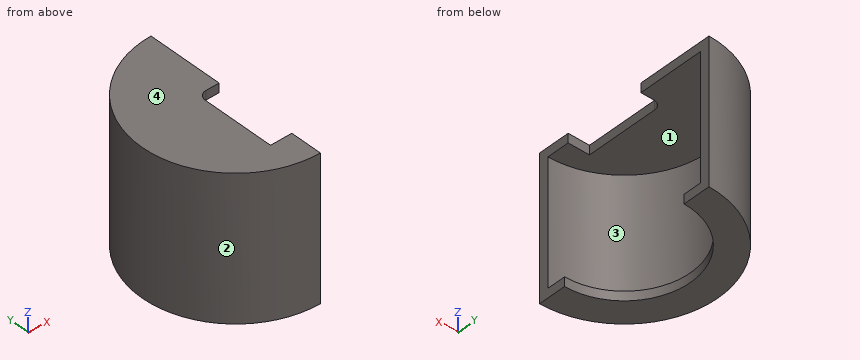
```python
from build123d import *

# Parameters (mm, degrees)
BOSS_EXTRU_1_DEPTH      = 34
BOSS_EXTRU_2_DEPTH      = 5
BOSS_EXTRU_3_DEPTH      = 5
ENL_V_MAT_EXTRU_1_DEPTH = 10


with BuildPart() as part:
    # Esquisse1 → Boss.-Extru.1 (new body, symmetric)
    with BuildSketch(Plane.XY):
        with BuildLine():
            Line((0, 51), (0, 46))
            ThreePointArc((0, 46), (-46, 0), (0, -46))
            Line((0, -46), (0, -51))
            ThreePointArc((0, -51), (-51, 0), (0, 51))
        make_face()
    extrude(amount=BOSS_EXTRU_1_DEPTH, both=True)

    # Esquisse2 → Boss.-Extru.2 (add)
    with BuildSketch(Plane.XY.offset(34)):
        with BuildLine():
            Line((0, 51), (0, -51))
            ThreePointArc((0, -51), (-51, 0), (0, 51))
        make_face()
    extrude(amount=BOSS_EXTRU_2_DEPTH)

    # Esquisse3 → Boss.-Extru.3 (add)
    with BuildSketch(Plane(origin=(0, 0, -34), x_dir=(-1, 0, 0), z_dir=(0, 0, -1))):
        with BuildLine():
            Line((0, 51), (0, 36))
            ThreePointArc((0, 36), (36, 0), (0, -36))
            Line((0, -36), (0, -51))
            ThreePointArc((0, -51), (51, 0), (0, 51))
        make_face()
    extrude(amount=BOSS_EXTRU_3_DEPTH)

    # Esquisse4 → Enlèv. mat.-Extru.1 (cut)
    with BuildSketch(Plane.XY.offset(39)):
        with BuildLine():
            Line((-11.59999996, 5.499999956), (-11.59999996, -2))
            Line((-11.59999996, -2), (-0.788986692, -2))
            ThreePointArc((-0.788986692, -2), (-2.112167134, 0.40155946), (0, 2.15))
            Line((0, 2.15), (0, 10.000000044))
            Line((0, 10.000000044), (-7.099999871, 10.000000044))
            ThreePointArc((-7.099999871, 10.000000044), (-10.281980449, 8.681980534), (-11.59999996, 5.499999956))
        make_face()
        with BuildLine():
            ThreePointArc((0, 2.15), (-2.112167134, 0.40155946), (-0.788986692, -2))
            Line((-0.788986692, -2), (0, -2))
            Line((0, -2), (0, 2.15))
        make_face()
        with BuildLine():
            Line((0, -2), (-0.788986692, -2))
            ThreePointArc((-0.788986692, -2), (-0.40155946, -2.112167134), (0, -2.15))
            Line((0, -2.15), (0, -2))
        make_face()
        with BuildLine():
            Line((0, 2.15), (0, -2))
            Line((0, -2), (0.788986692, -2))
            ThreePointArc((0.788986692, -2), (1.77747312, -1.209582286), (2.15, 0))
            ThreePointArc((2.15, 0), (1.52027958, 1.52027958), (0, 2.15))
        make_face()
        with BuildLine():
            Line((0.788986692, -2), (0, -2))
            Line((0, -2), (0, -2.15))
            ThreePointArc((0, -2.15), (0.40155946, -2.112167134), (0.788986692, -2))
        make_face()
        with BuildLine():
            Line((-0.788986692, -2), (-11.59999996, -2))
            Line((-11.59999996, -2), (-11.59999996, -33.8))
            Line((-11.59999996, -33.8), (0, -33.8))
            Line((0, -33.8), (0, -2.15))
            ThreePointArc((0, -2.15), (-0.40155946, -2.112167134), (-0.788986692, -2))
        make_face()
    extrude(amount=-ENL_V_MAT_EXTRU_1_DEPTH, mode=Mode.SUBTRACT)


solid = part.part
```
Model file for the job. Use its own axes, mm. Face numbers are marked on the shaded views. Give positions to 0.01 mm unless a question says otherwise; leave off trailing zeros. Loops run counter-clockwise (first coordinate to the right, second up) from the corner with the lowest first, then second, coordinate; pieces in that order, holes last. Notation, with made-up numbers: (48, -33) -> (57, -33) arc R10 ccw to (57, -28) -> close; hole circle Ø3 at (-21, 54.5). An arc over 180 degrees is marked (long way). Write each question's results on one line, items separated by ' | '.
(1) Cut at A-A on y = 31. List the corners of the cut face in (x, z), and give its area (3 significant figures).
Geometry results:
outline: (-40.5, -39) -> (-18.3, -39) -> (-18.3, -34) -> (-33.99, -34) -> (-33.99, 34) -> (0, 34) -> (0, 39) -> (-40.5, 39) -> close | area: 756 mm²
(2) Cut at C-C on z = -7. List the corners of the cut face in (x, y).
Geometry results:
outline: (0, -51) -> (0, -46) arc R46 cw to (0, 46) -> (0, 51) arc R51 ccw to start
(3) Probe line 1 along Z through (x, y) = (-20, -40.5); line 2 along Y through (x, z) = (-4, -33); line 3 along Z through (x, y) = (-17.5, 4.5). List the from-to ranges inside material, lowest first.
Geometry results:
line 1: z = -39 to -34, 34 to 39 | line 2: y = -50.84 to -45.83, 45.83 to 50.84 | line 3: z = 34 to 39
(4) Cut at D-D on y = 0. List the corners of the cut face in (x, z), and give its area (3 significant figures).
Geometry results:
outline: (-51, -39) -> (-36, -39) -> (-36, -34) -> (-46, -34) -> (-46, 34) -> (-11.6, 34) -> (-11.6, 39) -> (-51, 39) -> close | area: 612 mm²
(5) Cut at B-B on x = -29. List the corners of the cut face in (y, z), and give its area (3 significant figures).
Geometry results:
outline: (-41.95, -39) -> (-21.33, -39) -> (-21.33, -34) -> (-35.71, -34) -> (-35.71, 34) -> (35.71, 34) -> (35.71, -34) -> (21.33, -34) -> (21.33, -39) -> (41.95, -39) -> (41.95, 39) -> (-41.95, 39) -> close | area: 1,480 mm²
(6) Pull direction Y, two halves, no side cores. Call the marked faces 1, 2, 3 and 4: released by +Y, released by -Y, zero draft, split by the parting line, or undercut.
Geometry results:
face 1: undercut | face 2: split by the parting line | face 3: undercut | face 4: zero draft
(7) Flat gauge pins, fed straight in: pin 1 Ø4 at (y, z) = (23.5, 6.5) entering from +X; pin 2 Ø6 at (x, z) = (-13, 18.5) entering from -Y; pin 3 Ø4 at (x, z) = (-42.5, 15.5) entering from -Y; pin 4 Ø5.5 at (x, z) = (-2.5, 37.5) entering from -Y. Where does each tip first touch, or does it go through?
Geometry results:
pin 1: stops at x = -38.29 | pin 2: stops at y = -50.01 | pin 3: stops at y = -31 | pin 4: stops at y = -51
